The listing builds one solid part. Answer for the finished solid, in the listing's coordinates (mm). Round coordinates to 2 decimals unless told otherwise and drop trailing zeros. Loops run counter-clockwise (first coordinate to the right, second up) from the corner with the lowest first, then second, coordinate; pieces in that order, holes last. Notation, with made-up numbers: M 30.25,27.25 L 70.25,27.25 A6 cw 70.25,37.25 Z; hole C 12.5,12 d4. An arc over 180 degrees is marked long. Put each result on its own line as item: value. Start each with the question number.
(1) Section B-B, the plane z = -40 is taken. Determine the outline of the cut face in (x, y).
(2) Section C-C, the plane x = 34 is taken. Determine the outline of the cut face in (y, z).
(3) Straight lines are drawn through the part: line 1 (X direction, y = 8, z = -40); line 2 (X direction, y = 10.5, z = -13); line 3 (Y direction, x = 50, z = -25.5). For each, find the intervals that lie inside material, in ascending order.
(4) Section A-A, the plane x = 150 is taken. Determine the outline of the cut face in (y, z), then the cut area to 3 significant figures.
(5) A flat-ended cylindrical pin translates along its axis: P1, Ø6, axis at x = 105, z = -25.5, coming from the -Y side. Find the tip coordinate at first contact, or state that the pin passes through.
```python
from build123d import *

# Parameters (mm, degrees)
SKETCH1_W               = 200
SKETCH1_H               = 50
BOSS_EXTRUDE1_DEPTH     = 20
CUT_EXTRUDE1_DEPTH      = 30
CUT_EXTRUDE1_DEPTH_BACK = 221
SKETCH3_R               = 4.05
CUT_EXTRUDE2_DEPTH      = 67


with BuildPart() as part:
    # Sketch1 → Boss-Extrude1 (new body)
    with BuildSketch(Plane(origin=(0, 0, 0), x_dir=(1, 0, 0), z_dir=(0, 1, 0))):
        with Locations((100, 25)):
            Rectangle(SKETCH1_W, SKETCH1_H)
    extrude(amount=BOSS_EXTRUDE1_DEPTH)

    # Sketch2 → Cut-Extrude1 (cut, two sides: drawn at the far end of the back side and taken through both)
    with BuildSketch(Plane.ZY.offset(-CUT_EXTRUDE1_DEPTH_BACK)):
        with BuildLine():
            Line((-25, 20), (-28.5, 20))
            Line((-28.5, 20), (-28.5, 16.5))
            ThreePointArc((-28.5, 16.5), (-27.474873734, 18.974873734), (-25, 20))
        make_face()
        with BuildLine():
            ThreePointArc((-21.5, 16.5), (-22.525126266, 18.974873734), (-25, 20))
            Line((-25, 20), (-25, 13))
            ThreePointArc((-25, 13), (-22.525126266, 14.025126266), (-21.5, 16.5))
        make_face()
        with BuildLine():
            Line((-25, 13), (-25, 20))
            ThreePointArc((-25, 20), (-27.474873734, 18.974873734), (-28.5, 16.5))
            ThreePointArc((-28.5, 16.5), (-27.474873734, 14.025126266), (-25, 13))
        make_face()
        with BuildLine():
            Line((-21.5, 20), (-25, 20))
            ThreePointArc((-25, 20), (-22.525126266, 18.974873734), (-21.5, 16.5))
            Line((-21.5, 16.5), (-21.5, 20))
        make_face()
    extrude(amount=CUT_EXTRUDE1_DEPTH + CUT_EXTRUDE1_DEPTH_BACK, mode=Mode.SUBTRACT)

    # Sketch3 → Cut-Extrude2 (cut)
    with BuildSketch(Plane.XZ):
        with BuildLine():
            ThreePointArc((104.05, -10), (102.863782464, -7.136217536), (100, -5.95))
            Line((100, -5.95), (100, -14.05))
            ThreePointArc((100, -14.05), (102.863782464, -12.863782464), (104.05, -10))
        make_face()
        with BuildLine():
            Line((100, -14.05), (100, -5.95))
            ThreePointArc((100, -5.95), (95.95, -10), (100, -14.05))
        make_face()
        with BuildLine():
            ThreePointArc((54.05, -10), (52.863782464, -7.136217536), (50, -5.95))
            Line((50, -5.95), (50, -14.05))
            ThreePointArc((50, -14.05), (52.863782464, -12.863782464), (54.05, -10))
        make_face()
        with BuildLine():
            Line((50, -14.05), (50, -5.95))
            ThreePointArc((50, -5.95), (45.95, -10), (50, -14.05))
        make_face()
        with Locations(Location((50, -40, 0), (0, 0, 270))):
            Circle(SKETCH3_R)
        with Locations(Location((100, -40, 0), (0, 0, 270))):
            Circle(SKETCH3_R)
        with Locations(Location((150, -40, 0), (0, 0, 270))):
            Circle(SKETCH3_R)
        with Locations(Location((150, -10, 0), (0, 0, 270))):
            Circle(SKETCH3_R)
    extrude(amount=-CUT_EXTRUDE2_DEPTH, mode=Mode.SUBTRACT)


solid = part.part
```
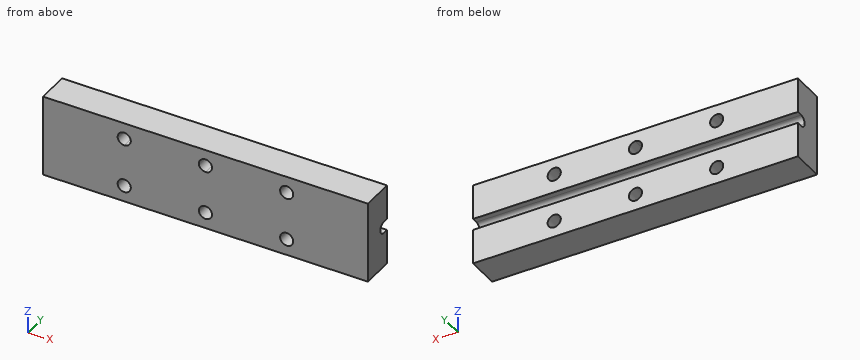
Recorded:
1. outline: M 0,0 L 45.95,0 L 45.95,20 L 0,20 Z; M 54.05,0 L 95.95,0 L 95.95,20 L 54.05,20 Z; M 104.05,0 L 145.95,0 L 145.95,20 L 104.05,20 Z; M 154.05,0 L 200,0 L 200,20 L 154.05,20 Z
2. outline: M 0,-50 L 20,-50 L 20,-28.5 L 16.5,-28.5 A3.5 cw 16.5,-21.5 L 20,-21.5 L 20,0 L 0,0 Z
3. line 1: x = 0 to 45.95, 54.05 to 95.95, 104.05 to 145.95, 154.05 to 200
3. line 2: x = 0 to 47.28, 52.72 to 97.28, 102.72 to 147.28, 152.72 to 200
3. line 3: y = 0 to 13.04
4. outline: M 0,-50 L 20,-50 L 20,-44.05 L 0,-44.05 Z; M 0,-35.95 L 20,-35.95 L 20,-28.5 L 16.5,-28.5 A3.5 cw 16.5,-21.5 L 20,-21.5 L 20,-14.05 L 0,-14.05 Z; M 0,-5.95 L 20,-5.95 L 20,0 L 0,0 Z
4. area: 632 mm²
5. P1: stops at y = 0
